The listing builds one solid part. Answer for the finished solid, in the listing's coordinates (mm). Round coordinates to 2 decimals unless told otherwise and drop trailing zeros. Loops run counter-clockwise (first coordinate to the right, second up) from the corner with the lowest first, then second, coordinate; pieces in that order, holes last. Notation, with made-up numbers: (66, -31) -> (101, -31) arc R17 ccw to (101, -14) -> close; hole circle Ø4 at (3.25, 69). An arc over 180 degrees is marked (long way). Use a Markdown table: item, result. Add a question column.
Q1. For a pull along X with two mould halves and no side action, classify faces 1 (the flat face through (45, 0, 0)), 2 (the flat face through (0, 0, 0)), 3 (the cylindrical face through (22.21, 2.5, 3.92)) as released by +X, released by -X, zero draft, split by the parting line, or undercut.
Q2. Given pin 1 Ø1.5 at (y, z) = (-3.5, 0.5) entering from -X; pin 2 Ø3 at (x, z) = (27.5, -2) entering from +Y; pin 3 Ø1 at (y, z) = (2, -2.5) entering from +X; pin 4 Ø5 at (x, z) = (23, 3.5) entering from -Y, each flat-ended and moving along its own axis, determine where each tip first touches the part or whether it passes through.
Q3. Consider line 1 (Y direction, x = 28.5, z = -0.25); line 2 (Y direction, x = 5.5, z = -1.5); line 3 (Z direction, x = 40, y = 0.75). Determine where each line is inside the solid, lowest interval first.
Q4. Section A-A on x = 39 is taken. Give the vertices of the cut face in (y, z).
from build123d import *

# Parameters (mm, degrees)
F0_R     = 4.65
F1_DEPTH = 45
F2_R     = 2
F3_R     = 2


with BuildPart() as f1:
    # F0 (on Right) → F1 (new body)
    with BuildSketch(Plane.YZ):
        Circle(F0_R)
    extrude(amount=F1_DEPTH)

    # F2
    f2_edges = [f1.edges().sort_by_distance(p)[0] for p in [
        (0, -4.65, 0),
    ]]
    fillet(f2_edges, radius=F2_R)

    # F3
    f3_edges = [f1.edges().sort_by_distance(p)[0] for p in [
        (45, -4.65, 0),
    ]]
    fillet(f3_edges, radius=F3_R)


solid = f1.part
Checked values:
| question | item | result |
|---|---|---|
| 1 | face 1 | released by +X |
| 1 | face 2 | released by -X |
| 1 | face 3 | zero draft |
| 2 | pin 1 | stops at x = 0 |
| 2 | pin 2 | stops at y = 4.62 |
| 2 | pin 3 | stops at x = 45 |
| 2 | pin 4 | stops at y = -4.54 |
| 3 | line 1 | y = -4.64 to 4.64 |
| 3 | line 2 | y = -4.4 to 4.4 |
| 3 | line 3 | z = -4.59 to 4.59 |
| 4 | outline | circle Ø9.3 at (0, 0) |
